```python
from build123d import *

# Parameters (mm, degrees)
SKETCH015_R     = 5
PAD004_DEPTH    = 135
POCKET012_DEPTH = 43
POCKET013_DEPTH = 43


with BuildPart() as part:
    # Sketch015 → Pad004 (new body)
    with BuildSketch(Plane.XZ):
        Circle(SKETCH015_R)
    extrude(amount=PAD004_DEPTH)

    # Sketch026 (on Face3 of Pad004) → Pocket012 (cut)
    with BuildSketch(Plane.XZ.offset(135)):
        Polygon((3.531062, -3.54), (3.531062, 3.54), (-3.531062, 3.54), (-3.87, 6.02), (6.78, 6.02), (6.88, -3.72), align=None)
    extrude(amount=-POCKET012_DEPTH, mode=Mode.SUBTRACT)

    # Sketch027 (on Face5 of Pocket012) → Pocket013 (cut)
    with BuildSketch(Plane.XZ.offset(135)):
        Polygon((-3.531062, 3.54), (-3.531062, -3.54), (3.531062, -3.54), (3.531062, -6.25), (-6.79, -6.25), (-6.79, 3.54), align=None)
    extrude(amount=-POCKET013_DEPTH, mode=Mode.SUBTRACT)


with BuildPart() as part_1:
    # Body005 placement: moved
    add(part.part.moved(Location((0, 23, 0))))


solid = part_1.part
```
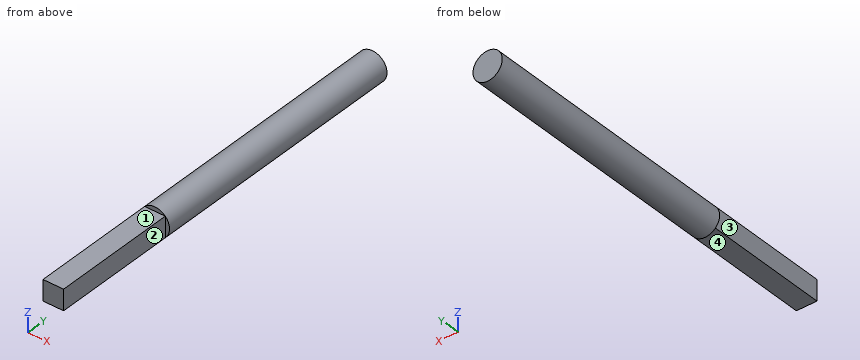
For this review, take the finished solid that the model builds, in its own axes (mm). Face numbers are marked on the shaded views. A direction names the side the tool comes from. Give positions to 0.01 mm unless a question says otherwise; leave off trailing zeros. Write each loop counter-clockwise with the first axis right and the second up, starting at its lowest first coordinate (ties: lowest second). Pieces come first, ordered by that corner, then holes. Notation, with made-up numbers: M 88.25,80.5 L 139.25,80.5 A11 cw 139.25,87.5 Z; hole C 39,5.25 d9. An arc over 180 degrees is marked long. One line per item, written item: value.
1) Take a section at A-A, the plane x = 0. Write out the cut boundary in (y, z), then the cut area to 3 significant figures.
Results are:
outline: M -112,-3.54 L -69,-3.54 L -69,-5 L 23,-5 L 23,5 L -69,5 L -69,3.54 L -112,3.54 Z
area: 1,220 mm²
2) For P1, Ø2, axis at y = -96.5, z = 0.5, coming from the -X side; P2, Ø3.5, axis at x = -0.5, y = -91, coming from the +Z side; P3, Ø1.6, axis at x = 1, z = 4.5, coming from the -Y side, all flat-tipped, find the tip position at first contact; note any pin that passes through.
Results are:
P1: stops at x = -3.53
P2: stops at z = 3.54
P3: stops at y = -69
3) Take a section at D-D, the plane y = -79. Write out the cut boundary in (x, z).
Results are:
outline: M -3.53,-3.54 L 3.53,-3.54 L 3.53,3.54 L -3.53,3.54 Z
4) For the marked faces 1, 2, 3 and 4, list the 3-axis set-ups (+Z, -Z, +X, -X, +Y, -Y) from which the entire face can be reached by the end or side of a thin tool; tool diameter is ignored.
Results are:
face 1: +Z, +X, -X, -Y
face 2: +Z, -Z, +X, -Y
face 3: +Z, -Z, -X, -Y
face 4: -Z, +X, -X, -Y
5) For line 1 (X direction, y = -69.5, z = 0.5); line 2 (Y direction, x = 4, z = -2.75); line 3 (Z direction, x = 3, y = -93.5), list the stretches that pass through material, from the lowest coordinate up. Write a range as from..to.
Results are:
line 1: x = -3.53..3.53
line 2: y = -69..23
line 3: z = -3.54..3.54
6) Take a section at B-B, the plane z = 0. Write out the cut boundary in (x, y), then the cut area to 3 significant figures.
Results are:
outline: M -5,-69 L -3.53,-69 L -3.53,-112 L 3.53,-112 L 3.53,-69 L 5,-69 L 5,23 L -5,23 Z
area: 1,220 mm²
7) Take a section at C-C, the plane y = 1.5. Write out the cut boundary in (x, z).
Results are:
outline: C 0,0 d10
